Autodesk Inventor part; units mm, degrees
ref_plane "YZ Plane" through (0, 0, 0) normal (1, 0, 0) x (0, 1, 0)
ref_plane "XZ Plane" through (0, 0, 0) normal (0, 1, 0) x (-1, 0, 0)
ref_plane "XY Plane" through (0, 0, 0) normal (0, 0, 1) x (1, 0, 0)
sketch "Sketch1" plane through (0, 0, 0) normal (0, 0, 1) x (1, 0, 0)
  line L0 (-44.9013, 44.9013) -> (44.9013, -44.9013)
  line L1 (-44.9013, 44.9013) -> (82.0987, 44.9013) construction
  line L2 (-44.9013, 44.9013) -> (-44.9013, 38.5513)
  line L3 (44.9013, -44.9013) -> (44.9013, -57.6013)
  line L4 (44.9013, -57.6013) -> (-44.9013, 38.5513)
  line L5 (44.9013, -57.6013) -> (44.9013, -76.6513) construction
  line L6 (-44.9013, 38.5513) -> (-44.9013, -76.6513) construction
  line L7 (-44.9013, 38.5513) -> (70.3013, 38.5513) construction
  line L8 (-44.9013, -76.6513) -> (44.9013, -76.6513)
  line L9 (-44.9013, -76.6513) -> (-44.9013, -83.0013)
  line L10 (44.9013, -76.6513) -> (44.9013, -83.0013)
  line L11 (44.9013, -76.6513) -> (51.2513, -76.6513) construction
  line L12 (-44.9013, -83.0013) -> (44.9013, -83.0013)
  line L13 (44.9013, -57.6013) -> (25.8513, -76.6513)
  line L14 (44.9013, -57.6013) -> (71.842, -57.6013) construction
  line L15 (44.9013, -57.6013) -> (37.9664, -50.1761) construction
  line L16 (37.9664, -50.1761) -> (11.4912, -76.6513)
  line L17 (37.9664, -50.1761) -> (75.408, -50.1761) construction
  point P0 (0, 0)
  point P1 (0, 0)
  dimension "d0" = 127
  dimension "d1" = 45
  dimension "d2" = 6.35
  dimension "d4" = 19.05
  dimension "d5" = 12.7
  dimension "d6" = 90
  dimension "d7" = 6.35
  dimension "d8" = 90
  dimension "d9" = 135
  dimension "d10" = 10.16
  dimension "d11" = 135
extrude "Extrusion1" add sketch "Sketch1" against normal blind 127
sketch "Sketch4" plane through (37.9664, -50.1761, -127) normal (-0.7308, -0.6826, 0) x (0, 0, 1)
  line L0 (0, -1.2778) -> (0, 0)
  line L1 (127, 0) -> (127, -1.2778)
  line L2 (0, 0) -> (127, 0) construction
  line L3 (127, 0) -> (0, 0)
  line L4 (63.5, 0) -> (63.5, 5.08) construction
  line L5 (63.5, 0) -> (68.58, 0) construction
  line L6 (53.975, 11.43) -> (73.025, 11.43)
  line L7 (73.025, 11.43) -> (73.025, 5.08)
  line L8 (73.025, 5.08) -> (53.975, 5.08)
  line L9 (53.975, 5.08) -> (53.975, 11.43)
  point P0 (127, 62.5845)
  dimension "d22" = 5.08
  dimension "d23" = 90
  dimension "d24" = 19.05
  dimension "d25" = 6.35
extrude "Extrusion4" cut sketch "Sketch4" against normal up to next
properties part number "proto_1b"
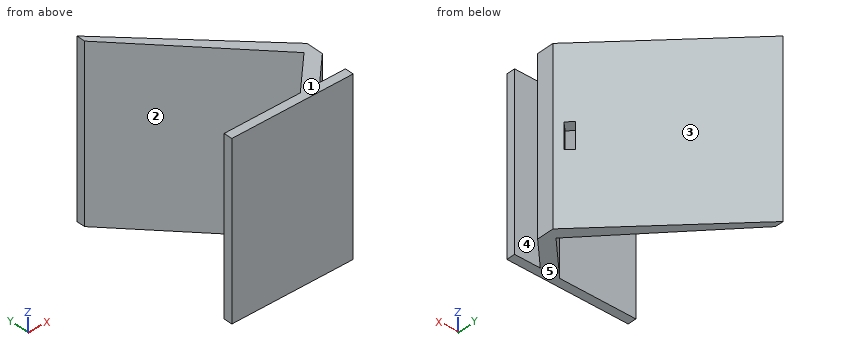
Here's how the part is built. I have some questions about the finished solid (model axes, mm). Face numbers are marked on the shaded views. A direction names the side the tool comes from. Give positions to 0.01 mm unless a question says otherwise; leave off trailing zeros. Order: outer loops, then holes, each group sorted by start corner. A loop starts at its lowest first (then second) coordinate and runs counter-clockwise, first axis right, second up. Notation, with made-up numbers: (-6.75, 40) -> (20.25, 40) arc R16 cw to (20.25, 48) -> close; hole circle Ø9 at (11, 14). An arc over 180 degrees is marked (long way). Use a Markdown table: item, result. Add a question column.
Item 1: Imagine slicing it at D-D on y = -28. Please give me the cut outline in (x, z), plus the area to 3 significant figures.
Item 2: If we mould it in two halves opening along Y, with no side actions, what happens to the marked faces 3, 4 and 5? For each: pulls with the +Y half, pulls with the -Y half, needs draft (parallel to the pull), parting line crosses it, or undercut.
Item 3: Imagine slicing it at A-A on x = -38. Please give me the cut outline in (y, z), plus the area to 3 significant figures.
Item 4: I need wall thicknesses on line 1 (Z direction, x = 34, y = -42.5) (3 decimals); line 2 (Y direction, x = 28.5, z = -112.5); line 3 (Y direction, x = 31, z = -67.5). Which ranges of each line are inside material? Lowest first, please.
Item 5: Will these pins go through, and if not, where does the flat tip stop? pin 1 (21 mm diameter, centred on x = 32, z = -93.5, fed in from +Y); pin 2 (1.5 mm diameter, centred on x = -15, z = -16.5, fed in from +Y); pin 3 (1.5 mm diameter, centred on y = -69, z = -47.5, fed in from -X).
Item 6: Imagine slicing it at B-B on z = -58.5. Please give me the cut outline in (x, y).
Item 7: Imagine slicing it at C-C on z = -117. Please give me the cut outline in (x, y), plus the area to 3 significant figures.
Item 8: For the marked faces 1 and 2, which set-ups out of +Z, -Z, +X, -X, +Y, -Y let a thin tool reach every point of the face, with its end or its side?
Data:
| question | item | result |
|---|---|---|
| 1 | outline | (17.25, -127) -> (28, -127) -> (28, 0) -> (17.25, 0) -> close |
| 1 | area | 1,360 mm² |
| 2 | face 3 | pulls with the +Y half |
| 2 | face 4 | undercut |
| 2 | face 5 | needs draft |
| 3 | outline | (-83, -127) -> (-76.65, -127) -> (-76.65, 0) -> (-83, 0) -> close; (31.16, -127) -> (38, -127) -> (38, 0) -> (31.16, 0) -> close |
| 3 | area | 1,670 mm² |
| 4 | line 1 | z = -127 to -73.025, -53.975 to 0 |
| 4 | line 2 | y = -83 to -76.65, -74 to -59.64, -40.04 to -28.5 |
| 4 | line 3 | y = -83 to -76.65, -71.5 to -57.14, -41.04 to -31 |
| 5 | pin 1 | stops at y = -21.5 |
| 5 | pin 2 | stops at y = 15.75 |
| 5 | pin 3 | stops at x = 18.39 |
| 6 | outline | (-44.9, -83) -> (44.9, -83) -> (44.9, -76.65) -> (25.85, -76.65) -> (44.9, -57.6) -> (44.9, -44.9) -> (40.69, -40.69) -> (34.5, -46.46) -> (37.97, -50.18) -> (11.49, -76.65) -> (-44.9, -76.65) -> close; (-44.9, 38.55) -> (30.16, -41.82) -> (36.19, -36.19) -> (-44.9, 44.9) -> close |
| 7 | outline | (-44.9, -83) -> (44.9, -83) -> (44.9, -76.65) -> (25.85, -76.65) -> (44.9, -57.6) -> (44.9, -44.9) -> (-44.9, 44.9) -> (-44.9, 38.55) -> (37.97, -50.18) -> (11.49, -76.65) -> (-44.9, -76.65) -> close |
| 7 | area | 1,750 mm² |
| 8 | face 1 | +Z, +X, -X, +Y, -Y |
| 8 | face 2 | +Z, -Z, -X |
